Study the drawing (mm; zero at the part's minimum x, y, z) and answer. A direction names the side the tool comes from. Round coordinates to 2 decimals unless told otherwise and drop trailing zeros. Loops run counter-clockwise (first coordinate to the right, second up) from the corner with the lowest first, then second, coordinate; pieces in that order, holes last. Notation, with made-up numbers: (-8, 1.25) -> (50, 1.25) arc R28 cw to (50, 37.25) -> close; hole circle Ø9 at (32, -36.5). An arc over 180 degrees is marked (long way). Answer in a Markdown table with one row per item. Add a question column.
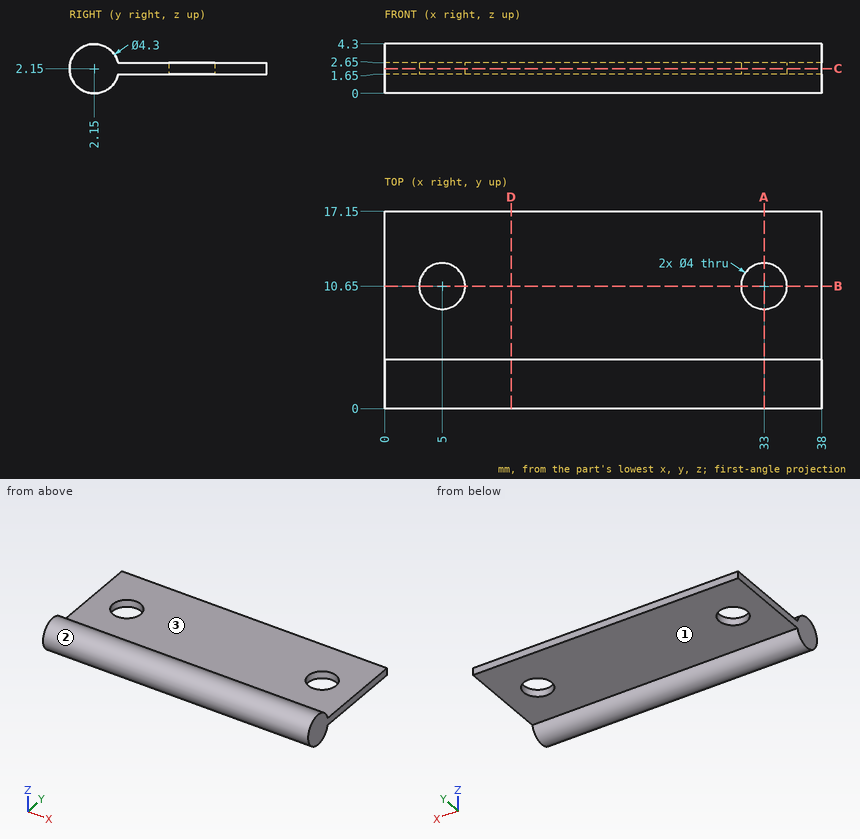
Item 1: Section B-B, the plane y = 10.65 is taken. Write down the section's boundary in (x, z), and give its area (3 significant figures).
Item 2: Section A-A, the plane x = 33 is taken. Write down the section's boundary in (y, z), and give its area (3 significant figures).
Item 3: A flat-ended cylindrical pin translates along its axis: P1, Ø4, axis at x = 22.5, y = 7.5, coming from the +Z side. Find the tip coordinate at first contact, or state that the pin passes through.
Item 4: For the marked faces 1, 2 and 3, determine the directions among +Z, -Z, +X, -X, +Y, -Y from which every point of the face is accessible in a straight line to the end or side of a thin tool.
Item 5: Consider L1, parallel to Y at x = 33, z = 2.2; L2, parallel to Z at x = 8.5, y = 8.25. Determine where each line is inside the solid, lowest interval first. Write a range as from..to.
Item 6: Section C-C, the plane z = 2.15 is taken. Write down the section's boundary in (x, y), and give its area (3 significant figures).
Item 7: Section D-D, the plane x = 11 is taken. Write down the section's boundary in (y, z).
Here are the results:
| question | item | result |
|---|---|---|
| 1 | outline | (0, 1.65) -> (3, 1.65) -> (3, 2.65) -> (0, 2.65) -> close; (7, 1.65) -> (31, 1.65) -> (31, 2.65) -> (7, 2.65) -> close; (35, 1.65) -> (38, 1.65) -> (38, 2.65) -> (35, 2.65) -> close |
| 1 | area | 30.0 mm² |
| 2 | outline | (4.24, 1.65) -> (8.65, 1.65) -> (8.65, 2.65) -> (4.24, 2.65) arc R2.15 ccw (long way) to start; (12.65, 1.65) -> (17.15, 1.65) -> (17.15, 2.65) -> (12.65, 2.65) -> close |
| 2 | area | 23.4 mm² |
| 3 | P1 | stops at z = 2.65 |
| 4 | face 1 | -Z, +X, -X, +Y |
| 4 | face 2 | +X, -X |
| 4 | face 3 | +Z, +X, -X, +Y |
| 5 | L1 | y = 0..8.65, 12.65..17.15 |
| 5 | L2 | z = 1.65..2.65 |
| 6 | outline | (0, 0) -> (38, 0) -> (38, 17.15) -> (0, 17.15) -> close; hole circle Ø4 at (5, 10.65); hole circle Ø4 at (33, 10.65) |
| 6 | area | 627 mm² |
| 7 | outline | (4.24, 1.65) -> (17.15, 1.65) -> (17.15, 2.65) -> (4.24, 2.65) arc R2.15 ccw (long way) to start |
